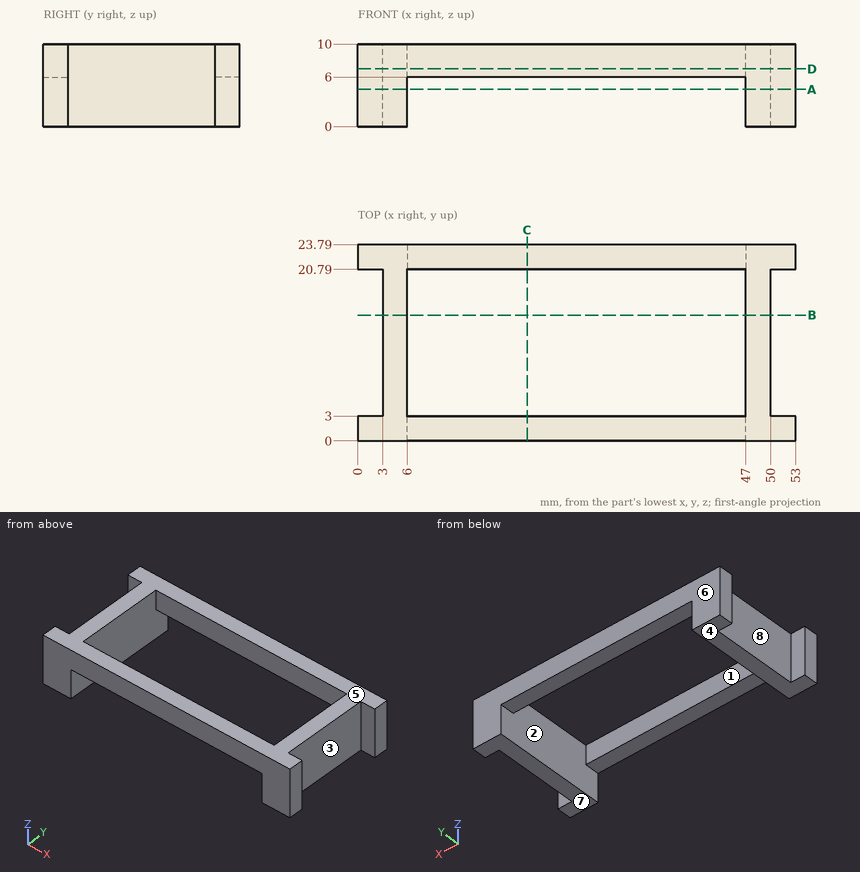
Input: dimensioned drawing with shaded views. Units: mm. Origin: part minimum x, y, z. A direction names the side the tool comes from. Coordinates: 2 decimals unless noted, no trailing zeros. Order: outer loops, then holes, each group sorted by start corner. A loop starts at its lowest first (then second) coordinate and runs counter-clockwise, first axis right, second up. Notation, with made-up numbers: (42, 26) - (74, 26) arc R11 cw to (74, 47) - close; hole circle Ø9 at (65.5, 25). An arc over 180 degrees is marked (long way). Return JSON: item names as keys, results as strings. Group by question number.
1. Cut plane C-C (x = 20.5). Output: boundary loops of the cut face in (y, z).
2. Cut plane B-B (y = 15.25). Output: boundary loops of the cut face in (x, z), plus the area to 3 significant figures.
3. Cut plane A-A (z = 4.5). Output: boundary loops of the cut face in (x, y), plus the area to 3 significant figures.
4. Set-up query: the marked faces 1, 2, 3, 4 and 5. Return all of +Z, -Z, +X, -X, +Y, -Y with unobstructed straight access to the full face (end or side cutting, diameter ignored); none if empty.
5. Cut plane D-D (z = 7). Output: boundary loops of the cut face in (x, y).
6. Material intervals for line 1 along Y through (x, z) = (14, 8); line 2 along X through (y, z) = (2.5, 2.5); line 3 along X through (y, z) = (6, 9.75), sorted ascending. Write a range as [from, to].
7. Pull-direction query (Y, two-part tool) for the marked faces 6, 7 and 8; classes: pulls with the +Y half, pulls with the -Y half, needs draft (parallel to the pull), parting line crosses it, or undercut.
8. Pin query (flat end, axial travel): pin 1 (1.5 mm diameter, centred on x = 36.5, y = 21.5, fed in from -Z); pin 2 (3 mm diameter, centred on y = 8.5, z = 5, fed in from +X); pin 3 (4 mm diameter, centred on x = 14, z = 4.5, fed in from -Y); pin 4 (3 mm diameter, centred on y = 15.5, z = 5, fed in from -X). Return the tip coordinate at first contact, or that it passes through.
Resolved:
{
 "1": {"outline": "(0, 6) - (3, 6) - (3, 10) - (0, 10) - close; (20.79, 6) - (23.79, 6) - (23.79, 10) - (20.79, 10) - close"},
 "2": {"outline": "(3, 0) - (6, 0) - (6, 10) - (3, 10) - close; (47, 0) - (50, 0) - (50, 10) - (47, 10) - close", "area": "60.0 mm²"},
 "3": {"outline": "(0, 0) - (6, 0) - (6, 23.79) - (0, 23.79) - (0, 20.79) - (3, 20.79) - (3, 3) - (0, 3) - close; (47, 0) - (53, 0) - (53, 3) - (50, 3) - (50, 20.79) - (53, 20.79) - (53, 23.79) - (47, 23.79) - close", "area": "179 mm²"},
 "4": {"face 1": "+Z, -Z", "face 2": "-Z", "face 3": "+Z, -Z, +X", "face 4": "-Z, +X, -X, +Y, -Y", "face 5": "+Z, +X, -X, +Y, -Y"},
 "5": {"outline": "(0, 0) - (53, 0) - (53, 3) - (50, 3) - (50, 20.79) - (53, 20.79) - (53, 23.79) - (0, 23.79) - (0, 20.79) - (3, 20.79) - (3, 3) - (0, 3) - close; hole (6, 3) - (47, 3) - (47, 20.79) - (6, 20.79) - close"},
 "6": {"line 1": "y = [0, 3], [20.79, 23.79]", "line 2": "x = [0, 6], [47, 53]", "line 3": "x = [3, 6], [47, 50]"},
 "7": {"face 6": "pulls with the +Y half", "face 7": "needs draft", "face 8": "undercut"},
 "8": {"pin 1": "stops at z = 6", "pin 2": "stops at x = 50", "pin 3": "stops at y = 0", "pin 4": "stops at x = 3"}
}
